Geometry: final body of the model. Coordinates: model frame, mm. Round coordinates to 2 decimals unless told otherwise and drop trailing zeros. Loops run counter-clockwise (first coordinate to the right, second up) from the corner with the lowest first, then second, coordinate; pieces in that order, holes last. Notation, with made-up numbers: M 70,49 L 114,49 A31 cw 114,73 Z; hole C 68,54 d4. An arc over 180 degrees is marked long. Answer as a JSON object with one key per item and string values.
from build123d import *

# Parameters (mm, degrees)
SKETCH1_W           = 86
SKETCH1_H           = 20
BOSS_EXTRUDE1_DEPTH = 1.3
SKETCH2_W           = 30
SKETCH2_H           = 1.4
SKETCH2_W_2         = 1.4
SKETCH2_H_2         = 10
BOSS_EXTRUDE2_DEPTH = 1.3
SKETCH3_W           = 1
SKETCH3_H           = 10
CUT_EXTRUDE1_DEPTH  = 46.858586982


with BuildPart() as part:
    # Sketch1 → Boss-Extrude1 (new body)
    with BuildSketch(Plane.XY):
        Rectangle(SKETCH1_W, SKETCH1_H)
    extrude(amount=BOSS_EXTRUDE1_DEPTH)

    # Sketch2 → Boss-Extrude2 (add)
    with BuildSketch(Plane.XY.offset(1.3)):
        with Locations((0, -10.7)):
            Rectangle(SKETCH2_W, SKETCH2_H)
        with Locations((-43.7, 0)):
            Rectangle(SKETCH2_W_2, SKETCH2_H_2)
        with Locations((43.7, 0)):
            Rectangle(SKETCH2_W_2, SKETCH2_H_2)
    extrude(amount=-BOSS_EXTRUDE2_DEPTH)

    # Sketch3 → Cut-Extrude1 (cut, through all)
    with BuildSketch(Plane.XY.offset(1.3)):
        with Locations((-10.5, 0.5)):
            Rectangle(SKETCH3_W, SKETCH3_H)
        with Locations((10.5, 0.5)):
            Rectangle(SKETCH3_W, SKETCH3_H)
    extrude(amount=-CUT_EXTRUDE1_DEPTH, mode=Mode.SUBTRACT)


solid = part.part
1) Section query B-B (z = 1.1). Return the cut outline in (x, y), and give its area (3 significant figures).
Results:
{"outline": "M -44.4,-5 L -43,-5 L -43,-10 L -15,-10 L -15,-11.4 L 15,-11.4 L 15,-10 L 43,-10 L 43,-5 L 44.4,-5 L 44.4,5 L 43,5 L 43,10 L -43,10 L -43,5 L -44.4,5 Z; hole M -11,-4.5 L -10,-4.5 L -10,5.5 L -11,5.5 Z; hole M 10,-4.5 L 11,-4.5 L 11,5.5 L 10,5.5 Z", "area": "1,770 mm2"}
2) Section query D-D (x = 34.5). Return the cut outline in (y, z), and give its area (3 significant figures).
Results:
{"outline": "M -10,0 L 10,0 L 10,1.3 L -10,1.3 Z", "area": "26.0 mm2"}
3) Pin query (flat end, axial travel): P1, Ø0.6, axis at x = -43.5, z = 1, coming from the +Y side; P2, Ø0.6, axis at y = 7, z = 1, coming from the -X side; P3, Ø0.6, axis at x = -43.5, z = 0.5, coming from the -Y side. Return the tip coordinate at first contact, or that it passes through.
Results:
{"P1": "y = 5", "P2": "x = -43", "P3": "y = -5"}
4) Ray query, line 1 (X direction, y = 0.5, z = 1.15); line 2 (Y direction, x = 29, z = 1.15); line 3 (X direction, y = 6.5, z = 0.55). Return the intervals inside material, ascending.
Results:
{"line 1": "-44.4 to -11, -10 to 10, 11 to 44.4", "line 2": "-10 to 10", "line 3": "-43 to 43"}
5) Section query A-A (y = 2.5). Return the cut outline in (x, z).
Results:
{"outline": "M -44.4,0 L -11,0 L -11,1.3 L -44.4,1.3 Z; M -10,0 L 10,0 L 10,1.3 L -10,1.3 Z; M 11,0 L 44.4,0 L 44.4,1.3 L 11,1.3 Z"}
6) Section query C-C (y = 8.5). Return the cut outline in (x, z), and give its area (3 significant figures).
Results:
{"outline": "M -43,0 L 43,0 L 43,1.3 L -43,1.3 Z", "area": "112 mm2"}
